```python
from build123d import *

# Parameters (mm, degrees)
F0_W     = 215.526138
F0_H     = 254
F1_DEPTH = 6.35
F3_DEPTH = 254.001
F5_DEPTH = 25.4


with BuildPart() as f1:
    # F0 (on Front) → F1 (new body)
    with BuildSketch(Plane.XZ):
        Rectangle(F0_W, F0_H)
    extrude(amount=F1_DEPTH)

    # F2 (on face) → F3 (cut, through all)
    with BuildSketch(Plane.XY.offset(127)):
        Polygon((-107.763069, 0), (-107.763069, -6.35), (-101.413069, -6.35), align=None)
        Polygon((107.763069, 0), (101.413069, -6.35), (107.763069, -6.35), align=None)
    extrude(amount=-F3_DEPTH, mode=Mode.SUBTRACT)

    # F4 (on face) → F5 (cut)
    with BuildSketch(Plane(origin=(0, 0, 0), x_dir=(-1, 0, 0), z_dir=(0, 1, 0))):
        Polygon((88.9, 0), (0, 0), (-88.9, 0), (-88.9, -127), (88.9, -127), align=None)
    extrude(amount=-F5_DEPTH, mode=Mode.SUBTRACT)


solid = f1.part
```
Work out the finished part from the listing and answer in its coordinate system (mm). A direction names the side the tool comes from. Coordinates: 2 decimals unless noted, no trailing zeros. Order: outer loops, then holes, each group sorted by start corner. A loop starts at its lowest first (then second) coordinate and runs counter-clockwise, first axis right, second up. Notation, with made-up numbers: (24.25, 54) - (38.25, 54) arc R22 cw to (38.25, 74) - close; hole circle Ø8 at (-36, 59.25). An arc over 180 degrees is marked (long way). Answer as a JSON object with one key per item and string values.
1. Find section C-C on x = 2. Determine the outline of the cut face in (y, z).
Output values:
{"outline": "(-6.35, 0) - (0, 0) - (0, 127) - (-6.35, 127) - close"}
2. Consider line 1 (X direction, y = -5.25, z = -92); line 2 (X direction, y = -0.5, z = -41); line 3 (Z direction, x = -56, y = -1.25). Determine where each line is inside the solid, lowest interval first.
Output values:
{"line 1": "x = -102.51 to -88.9, 88.9 to 102.51", "line 2": "x = -107.26 to -88.9, 88.9 to 107.26", "line 3": "z = 0 to 127"}
3. Find section D-D on z = 111. Determine the outline of the cut face in (x, y).
Output values:
{"outline": "(-107.76, 0) - (-101.41, -6.35) - (101.41, -6.35) - (107.76, 0) - close"}
4. Find section A-A on z = -68. Determine the outline of the cut face in (x, y), plus the area to 3 significant figures.
Output values:
{"outline": "(-107.76, 0) - (-101.41, -6.35) - (-88.9, -6.35) - (-88.9, 0) - close; (88.9, -6.35) - (101.41, -6.35) - (107.76, 0) - (88.9, 0) - close", "area": "199 mm²"}
5. The mould has two halves that part along X. Classify faces 3 (the face through (-1, -3, 0)), 4 (the face through (-88.9, -3, -64)), 5 (the face through (-96, -3, -127)), 6 (the face through (104.633, -3.131, 1.778)): +X half, -X half, draft (parallel to the pull), parting line (faces both ways), or undercut.
Output values:
{"face 3": "undercut", "face 4": "undercut", "face 5": "draft", "face 6": "+X half"}
6. Find section B-B on y = -4.5. Determine the outline of the cut face in (x, z).
Output values:
{"outline": "(-103.26, -127) - (-88.9, -127) - (-88.9, 0) - (88.9, 0) - (88.9, -127) - (103.26, -127) - (103.26, 127) - (-103.26, 127) - close"}
7. A tool of negligible diameter and unlimited length cuts with its end or side. For faces 1 (the face through (88.9, -3, -63)), 2 (the face through (-2, -3, 127)), from which of +Z, -Z, +X, -X, +Y, -Y can it reach the whole face along a straight path? Write none if from no direction.
Output values:
{"face 1": "-Z, +Y, -Y", "face 2": "+Z, +X, -X, +Y, -Y"}
8. Each of these flat-tipped pins is pushed along its axis until it touches: P1, Ø3, axis at y = -2, z = -34.5, coming from the -X side; P2, Ø1, axis at x = -25.5, y = -4, coming from the -Z side; P3, Ø1, axis at y = -2.5, z = 73, coming from the +X side. Where does it stop, or does it pass through?
Output values:
{"P1": "stops at x = -107.26", "P2": "stops at z = 0", "P3": "stops at x = 105.76"}
